```python
from build123d import *

# Parameters (mm, degrees)
SKETCH040_R     = 1.6
PAD023_DEPTH    = 3
SKETCH041_W     = 10
SKETCH041_H     = 10
POCKET016_DEPTH = 3.001
CHAMFER005_SIZE = 3


with BuildPart() as part:
    # Sketch040 → Pad023 (new body)
    with BuildSketch(Plane.YZ):
        Polygon((41, -16.2), (41, 29.8), (-32.652229, 29.8), (-39, -6.2), (-39, -16.2), align=None)
        with Locations((36, 19.8)):
            Circle(SKETCH040_R, mode=Mode.SUBTRACT)
        with Locations((-29.338365, 19.8)):
            Circle(SKETCH040_R, mode=Mode.SUBTRACT)
        with Locations((21, -11.2)):
            Circle(SKETCH040_R, mode=Mode.SUBTRACT)
        with Locations((-11, -11.2)):
            Circle(SKETCH040_R, mode=Mode.SUBTRACT)
        with Locations((5, 7.5)):
            Circle(SKETCH040_R, mode=Mode.SUBTRACT)
        with Locations((26, 7.5)):
            Circle(SKETCH040_R, mode=Mode.SUBTRACT)
        with Locations((36, 3.8)):
            Circle(SKETCH040_R, mode=Mode.SUBTRACT)
    extrude(amount=PAD023_DEPTH)

    # Sketch041 → Pocket016 (cut, through all)
    with BuildSketch(Plane.YZ):
        with Locations((36, -11.2)):
            Rectangle(SKETCH041_W, SKETCH041_H)
        with BuildLine():
            Line((-39, -16.2), (-39, 3.8))
            Line((-39, 3.8), (-34, 3.8))
            ThreePointArc((-19, -11.2), (-23.393398, -0.593398), (-34, 3.8))
            Line((-19, -16.2), (-19, -11.2))
            Line((-39, -16.2), (-19, -16.2))
        make_face()
    extrude(amount=POCKET016_DEPTH, mode=Mode.SUBTRACT)

    # Chamfer005
    chamfer005_edges = [part.edges().sort_by_distance(p)[0] for p in [
        (1.5, -32.652229, 29.8),
        (1.5, -37.23673, 3.8),
        (1.5, -19, -16.2),
        (1.5, 41, 29.8),
        (1.5, 41, -6.2),
        (1.5, 31, -16.2),
    ]]
    chamfer(chamfer005_edges, length=CHAMFER005_SIZE)


with BuildPart() as part_1:
    # Body023 placement: moved
    add(part.part.moved(Location((40, 0, 0))))


solid = part_1.part
```
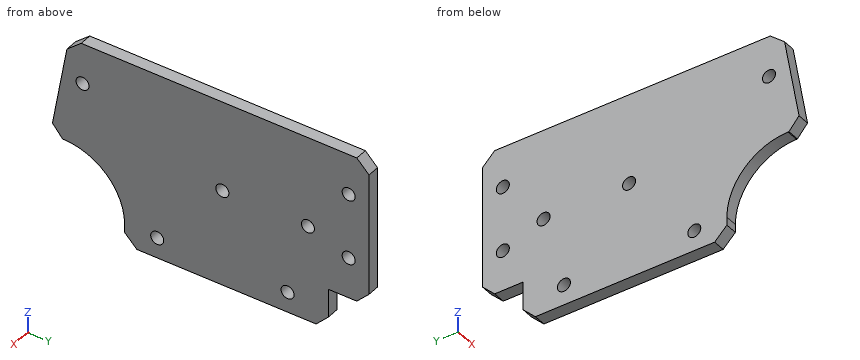
Can you work these out from the model? Positions are in its coordinate system, mm. Coordinates: 2 decimals unless noted, no trailing zeros. Loops run counter-clockwise (first coordinate to the right, second up) from the corner with the lowest first, then second, coordinate; pieces in that order, holes last.
1) Imagine slicing it at D-D on z = 19.8. List the corners of the cut face in (x, y) for me.
2) Imagine slicing it at C-C on x = 41.15. List the corners of the cut face in (y, z) for me.
3) Imagine slicing it at A-A on y = 36. List the corners of the cut face in (x, z) for me, plus the area to 3 significant figures.
4) I need wall thicknesses on probe 1 along Z at (x, y) = (42.4, 36); probe 2 along Y at (x, z) = (41.5, -11); probe 3 along Z at (x, y) = (40.95, 26). Which ranges of each line are inside material? Lowest first, please.
5) Imagine slicing it at B-B on y = 26. List the corners of the cut face in (x, z) for me.
6) For pin 1 (3 mm diameter, centred on y = 26, z = 7.5, fed in from +X); pin 2 (1 mm diameter, centred on x = 41, y = -22, fed in from -Z); pin 3 (0.9 mm diameter, centred on x = 42, y = 35.5, fed in from -Z); pin 4 (1 mm diameter, centred on x = 41.5, z = -8, fed in from +Y), each with a flat end and sliding along its axis, tell me the tip position at first contact or that it passes through.
Completed:
1. outline: (40, -34.42) - (43, -34.42) - (43, -30.94) - (40, -30.94) - close; (40, -27.74) - (43, -27.74) - (43, 34.4) - (40, 34.4) - close; (40, 37.6) - (43, 37.6) - (43, 41) - (40, 41) - close
2. outline: (-36.72, 6.75) - (-34.24, 3.8) - (-34, 3.8) arc R15 cw to (-19, -11.2) - (-19, -13.2) - (-16, -16.2) - (28, -16.2) - (31, -13.2) - (31, -6.2) - (38, -6.2) - (41, -3.2) - (41, 26.8) - (38, 29.8) - (-29.65, 29.8) - (-33.17, 26.85) - close; hole circle Ø3.2 at (-29.34, 19.8); hole circle Ø3.2 at (-11, -11.2); hole circle Ø3.2 at (5, 7.5); hole circle Ø3.2 at (21, -11.2); hole circle Ø3.2 at (26, 7.5); hole circle Ø3.2 at (36, 3.8); hole circle Ø3.2 at (36, 19.8)
3. outline: (40, -6.2) - (43, -6.2) - (43, 2.2) - (40, 2.2) - close; (40, 5.4) - (43, 5.4) - (43, 18.2) - (40, 18.2) - close; (40, 21.4) - (43, 21.4) - (43, 29.8) - (40, 29.8) - close
3. area: 88.8 mm2
4. probe 1: z = -6.2 to 2.2, 5.4 to 18.2, 21.4 to 29.8
4. probe 2: y = -19 to -12.59, -9.41 to 19.41, 22.59 to 31
4. probe 3: z = -16.2 to 5.9, 9.1 to 29.8
5. outline: (40, -16.2) - (43, -16.2) - (43, 5.9) - (40, 5.9) - close; (40, 9.1) - (43, 9.1) - (43, 29.8) - (40, 29.8) - close
6. pin 1: passes through
6. pin 2: stops at z = -2.91
6. pin 3: stops at z = -6.2
6. pin 4: stops at y = 31
